Here's how the part is built. I have some questions about the finished solid (model axes, mm). A direction names the side the tool comes from. Round coordinates to 2 decimals unless told otherwise and drop trailing zeros. Write each loop counter-clockwise with the first axis right and the second up, starting at its lowest first coordinate (ties: lowest second). Pieces come first, ordered by that corner, then holes. Notation, with made-up numbers: M 11,27.25 L 16,27.25 A18 cw 16,61.25 Z; hole C -2,58.5 d2. An arc over 180 degrees is marked long. Write item = value, one per line. Start each with the question number.
(1) I need wall thicknesses on line 1 along Z through (x, y) = (22.25, 8.25); line 2 along Z through (x, y) = (12.25, 10); line 3 along Z through (x, y) = (27, 16.75). Which ranges of each line are inside material? Lowest first, please.
(2) On a 3-axis mill with a long thin cutter (end or side, diameter ignored), from which of +Z, -Z, +X, -X, +Y, -Y can I reach the whole of each face in a straight line? I mean faces 1 (the flat face through (7.251, 9.714, 1.615)), 2 (the flat face through (18.475, 12, 2)), 3 (the cylindrical face through (15, 20, 4.5)). Say none if no direction works.
(3) If we mould it in two halves opening along X, with no side actions, what happens to faces 4 (the flat face through (7, 19, 0)), 5 (the flat face through (23.225, 12, 2)), 6 (the cylindrical face through (15.33, 4.76, 4.51))? For each: released by +X, released by -X, zero draft, split by the parting line, or undercut.
(4) Will these pins go through, and if not, where does the flat tip stop? pin 1 Ø1.2 at (y, z) = (6.5, 1.5) entering from -X; pin 2 Ø0.9 at (x, y) = (12, 14.5) entering from -Z; pin 3 Ø2 at (y, z) = (11, 1.5) entering from +X.
(5) I want a section at D-D (x = 21.5). List the corners of the cut face in (y, z) for me (1 decimal).
(6) I want a section at A-A (x = 27.25). List the corners of the cut face in (y, z) for me, and give its area (3 significant figures).
(7) I want a section at B-B (y = 3.75). Give the number of separate pieces and of enclosed holes in the cut face, and give its area (3 significant figures).
(8) I want a section at C-C (x = 10). List the corners of the cut face in (y, z) for me (3 decimals), and give its area (3 significant figures).
```python
from build123d import *

# Parameters (mm, degrees)
SKETCH_W             = 28
SKETCH_H             = 22
PAD002_DEPTH         = 5
POCKET001_DEPTH      = 0.8
SKETCH002_W          = 0.6
SKETCH002_H          = 23
POCKET_DEPTH         = 4
LINEARPATTERN_COUNT  = 9
LINEARPATTERN_PITCH  = 2.375
POCKET002_DEPTH      = 3.5
SKETCH006_W          = 28
SKETCH006_H          = 22
POCKET005_DEPTH      = 1
POCKET005_DEPTH_BACK = 1
PAD_DEPTH            = 2


with BuildPart() as part:
    # Sketch → Pad002 (new body)
    with BuildSketch(Plane.XY):
        with Locations((15, 12)):
            Rectangle(SKETCH_W, SKETCH_H)
    extrude(amount=PAD002_DEPTH)

    # Sketch001 → Pocket001 (cut)
    with BuildSketch(Plane.XY):
        with BuildLine():
            ThreePointArc((17.967868, 19.714572), (14.962963, 20.499886), (11.967982, 19.677535))
            Line((11.967982, 19.677535), (4.036475, 13.531422))
            ThreePointArc((4.036475, 13.531422), (3.750333, 12.536475), (4, 11.531754))
            Line((4, 11.531754), (12.33, 4.876817))
            ThreePointArc((12.33, 4.876817), (15.374304, 4.261687), (18.318313, 5.25112))
            Line((18.318313, 5.25112), (26, 11.531754))
            ThreePointArc((26, 11.531754), (26.249667, 12.536475), (25.963525, 13.531422))
            Line((25.963525, 13.531422), (17.967868, 19.714572))
        make_face()
    extrude(amount=POCKET001_DEPTH, mode=Mode.SUBTRACT)

    # Sketch002 → Pocket (cut)
    with BuildSketch(Plane.XY):
        with Locations((6.3, 11.5)):
            Rectangle(SKETCH002_W, SKETCH002_H)
    pocket = extrude(amount=POCKET_DEPTH, mode=Mode.SUBTRACT)

    # LinearPattern: Pocket ×9
    with Locations(*[(i * LINEARPATTERN_PITCH, 0, 0) for i in range(1, LINEARPATTERN_COUNT)]):
        add(pocket, mode=Mode.SUBTRACT)

    # Sketch003 → Pocket002 (cut)
    with BuildSketch(Plane(origin=(0.5, 0, 4), x_dir=(0.707107, 0, -0.707107), z_dir=(0.707107, 0, 0.707107))):
        with BuildLine():
            ThreePointArc((17.966363, 19.215428), (14.961232, 19.999875), (11.966488, 19.17666))
            Line((11.966488, 19.17666), (4.036475, 13.531422))
            ThreePointArc((4.036475, 13.531422), (3.750333, 12.536475), (4, 11.531754))
            Line((4, 11.531754), (12.33, 5.376817))
            ThreePointArc((12.33, 5.376817), (15.374304, 4.761687), (18.318313, 5.75112))
            Line((18.318313, 5.75112), (26, 11.531754))
            ThreePointArc((26, 11.531754), (26.249667, 12.536475), (25.963525, 13.531422))
            Line((25.963525, 13.531422), (17.966363, 19.215428))
        make_face()
    extrude(amount=POCKET002_DEPTH, mode=Mode.SUBTRACT)

    # Sketch006 → Pocket005 (cut, two sides)
    with BuildSketch(Plane.XY.offset(5)) as pocket005_sk:
        with Locations((15, 12)):
            Rectangle(SKETCH006_W, SKETCH006_H)
        with BuildLine():
            ThreePointArc((17.966363, 19.215428), (14.961232, 19.999875), (11.966488, 19.17666))
            Line((11.966488, 19.17666), (4.036475, 13.531422))
            ThreePointArc((4.036475, 13.531422), (3.750333, 12.536475), (4, 11.531754))
            Line((4, 11.531754), (12.33, 5.376817))
            ThreePointArc((12.33, 5.376817), (15.374304, 4.761687), (18.318313, 5.75112))
            Line((18.318313, 5.75112), (26, 11.531754))
            ThreePointArc((26, 11.531754), (26.249667, 12.536475), (25.963525, 13.531422))
            Line((25.963525, 13.531422), (17.966363, 19.215428))
        make_face(mode=Mode.SUBTRACT)
    extrude(amount=-POCKET005_DEPTH, mode=Mode.SUBTRACT)
    extrude(pocket005_sk.sketch, amount=POCKET005_DEPTH_BACK, mode=Mode.SUBTRACT)

    # Sketch004 → Pad (join)
    with BuildSketch(Plane.XY.offset(5)):
        Polygon((5, 19.805), (25, 19.805), (25, 15), (30, 15), (30, 10), (25, 10), (25, 4.805), (5, 4.805), (5, 10), (0, 10), (0, 15), (5, 15), align=None)
    extrude(amount=PAD_DEPTH)


solid = part.part
```
Returned:
q1.line_1 = 0 to 4, 5 to 7
q1.line_2 = 0.8 to 7
q1.line_3 = 0 to 4
q2.face_1 = -Z
q2.face_2 = -Z, +Y, -Y
q2.face_3 = +Y
q3.face_4 = zero draft
q3.face_5 = undercut
q3.face_6 = split by the parting line
q4.pin_1 = 1
q4.pin_2 = 0.8
q4.pin_3 = 29
q5.outline = M 1,0 L 7.9,0 L 7.9,0.8 L 17,0.8 L 17,0 L 23,0 L 23,4 L 16.7,4 L 16.7,5 L 19.8,5 L 19.8,7 L 4.8,7 L 4.8,5 L 8.1,5 L 8.1,4 L 1,4 Z
q6.outline = M 1,0 L 23,0 L 23,4 L 1,4 Z; M 10,5 L 15,5 L 15,7 L 10,7 Z
q6.area = 98.0 mm²
q7.separate_pieces = 10
q7.enclosed_holes = 0
q7.area = 90.4 mm²
q8.outline = M 1,0 L 6.738,0 L 6.738,0.8 L 18.153,0.8 L 18.153,0 L 23,0 L 23,4 L 17.777,4 L 17.777,5 L 19.805,5 L 19.805,7 L 4.805,7 L 4.805,5 L 7.098,5 L 7.098,4 L 1,4 Z
q8.area = 120 mm²
